```python
from build123d import *

# Parameters (mm, degrees)
SKETCH1_W                                       = 140
SKETCH1_H                                       = 140
BOSS_EXTRUDE1_DEPTH                             = 5
CSK_FOR_M3_FLAT_HEAD_MACHINE_SCREW1_D           = 3
CSK_FOR_M3_FLAT_HEAD_MACHINE_SCREW1_CSINK_D     = 8
CSK_FOR_M3_FLAT_HEAD_MACHINE_SCREW1_CSINK_ANGLE = 90


with BuildPart() as part:
    # Sketch1 → Boss-Extrude1 (new body)
    with BuildSketch(Plane.XY):
        with Locations((70, 70)):
            Rectangle(SKETCH1_W, SKETCH1_H)
    extrude(amount=BOSS_EXTRUDE1_DEPTH)

    # CSK for M3 Flat Head Machine Screw1 (through all)
    with Locations(Plane(origin=(0, 0, 0), x_dir=(-1, 0, 0), z_dir=(0, 0, -1))):
        with Locations((-130, 92), (-130, 48), (-10, 92), (-10, 48)):
            CounterSinkHole(CSK_FOR_M3_FLAT_HEAD_MACHINE_SCREW1_D / 2, CSK_FOR_M3_FLAT_HEAD_MACHINE_SCREW1_CSINK_D / 2, counter_sink_angle=CSK_FOR_M3_FLAT_HEAD_MACHINE_SCREW1_CSINK_ANGLE)


solid = part.part
```
Source: CAD feature listing. Evaluate the final solid. Frame: model axes, mm. Give positions to 0.01 mm unless a question says otherwise; leave off trailing zeros. Put each result on its own line as item: value. Start each with the question number.
1) Contact query for flat-ended pins moving along their axis: P1, Ø4, axis at x = 130, y = 48, coming from the -Z side; P2, Ø1.8, axis at x = 10, y = 92, coming from the +Z side. Output: stop coordinate, or through.
2) Draft query along Y for faces 1 (the face through (69, 71, 5)), 2 (the face through (69, 140, 2)), 3 (the face through (9.805, 93.487, 3.768)), 4 (the face through (69, 0, 2)). Return one class per face: released by +Y, released by -Y, zero draft, split by the parting line, or undercut.
3) Material intervals for probe 1 along X at (y, z) = (48, 3); probe 2 along Y at (x, z) = (130, 3.4); probe 3 along Y at (x, z) = (129, 2.15), sorted ascending.
Results are:
1. P1: stops at z = 2
1. P2: passes through
2. face 1: zero draft
2. face 2: released by +Y
2. face 3: undercut
2. face 4: released by -Y
3. probe 1: x = 0 to 8.5, 11.5 to 128.5, 131.5 to 140
3. probe 2: y = 0 to 46.5, 49.5 to 90.5, 93.5 to 140
3. probe 3: y = 0 to 46.44, 49.56 to 90.44, 93.56 to 140
